Verification items for the finished model (mm, model axes). Face numbers are marked on the shaded views. Round coordinates to 2 decimals unless told otherwise and drop trailing zeros. Write each loop counter-clockwise with the first axis right and the second up, starting at its lowest first coordinate (ties: lowest second). Pieces come first, ordered by that corner, then holes.
from build123d import *

# Parameters (mm, degrees)
SKETCH_1_R      = 12
SKETCH_1_R_2    = 1.7
SKETCH_1_R_3    = 1.6
EXTRUDE_1_DEPTH = 2
SKETCH_2_R      = 2.5
EXTRUDE_2_DEPTH = 15


with BuildPart() as part:
    # 草图1 → 凸台-拉伸1 (new body)
    with BuildSketch(Plane(origin=(0, 0, 0), x_dir=(1, 0, 0), z_dir=(0, 1, 0))):
        Circle(SKETCH_1_R)
        with Locations((-8, 0)):
            Circle(SKETCH_1_R_2, mode=Mode.SUBTRACT)
        with Locations((0, 8)):
            Circle(SKETCH_1_R_3, mode=Mode.SUBTRACT)
        with Locations((8, 0)):
            Circle(SKETCH_1_R_2, mode=Mode.SUBTRACT)
        with Locations((0, -8)):
            Circle(SKETCH_1_R_3, mode=Mode.SUBTRACT)
    extrude(amount=EXTRUDE_1_DEPTH)

    # 草图2 → 凸台-拉伸2 (add)
    with BuildSketch(Plane(origin=(0, 2, 0), x_dir=(1, 0, 0), z_dir=(0, 1, 0))):
        Circle(SKETCH_2_R)
    extrude(amount=EXTRUDE_2_DEPTH)


solid = part.part
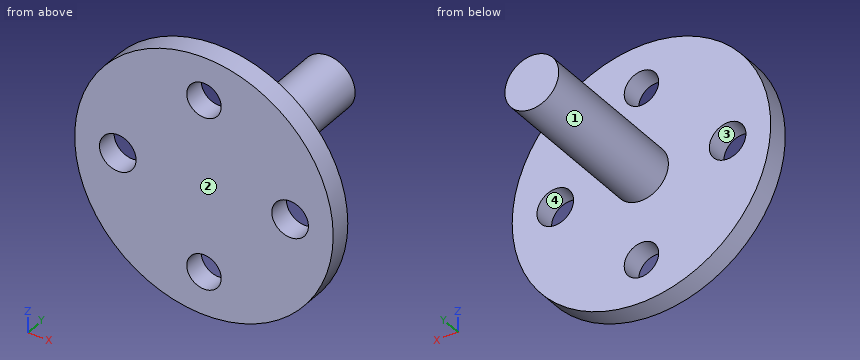
Q1. Release check for a two-part mould opening along Z. For the marked faces 1, 2, 3 and 4 record: released by +Z, released by -Z, zero draft, split by the parting line, or undercut.
Recorded:
face 1: split by the parting line
face 2: zero draft
face 3: undercut
face 4: undercut
Q2. Sectioned sample at D-D (z = -8). Enter the section's corners in (x, y), plus the area to 3 significant figures.
Recorded:
outline: (-8.94, 0) - (-1.6, 0) - (-1.6, 2) - (-8.94, 2) - close; (1.6, 0) - (8.94, 0) - (8.94, 2) - (1.6, 2) - close
area: 29.4 mm2
Q3. Material ranges on line 1 along X through (y, z) = (1.55, 0); line 2 along Z through (x, y) = (0, 1.35); line 3 along Z through (x, y) = (0.5, 1), recorded low to high.
Recorded:
line 1: x = -12 to -9.7, -6.3 to 6.3, 9.7 to 12
line 2: z = -12 to -9.6, -6.4 to 6.4, 9.6 to 12
line 3: z = -11.99 to -9.52, -6.48 to 6.48, 9.52 to 11.99
Q4. Sectioned sample at B-B (z = -0.5). Enter the section's corners in (x, y), plus the area to 3 significant figures.
Recorded:
outline: (-11.99, 0) - (-9.62, 0) - (-9.62, 2) - (-11.99, 2) - close; (-6.38, 0) - (6.38, 0) - (6.38, 2) - (2.45, 2) - (2.45, 17) - (-2.45, 17) - (-2.45, 2) - (-6.38, 2) - close; (9.62, 0) - (11.99, 0) - (11.99, 2) - (9.62, 2) - close
area: 108 mm2
Q5. Depth check by flat-ended pin: P1, Ø1, axis at x = -7, z = -3.5, coming from the -Y side; P2, Ø4, axis at y = 2.5, z = 2.5, coming from the +X side; P3, Ø1.5, axis at x = -1.5, z = -7.5, coming from the +Y side; P4, Ø5, axis at x = 3.5, y = 11, coming from the -Z side. Enter the tip coordinate at first touch or a pass-through.
Recorded:
P1: stops at y = 0
P2: stops at x = 11.99
P3: stops at y = 2
P4: stops at z = -2.29
Q6. Sectioned sample at A-A (x = 0). Enter the section's corners in (y, z), plus the area to 3 significant figures.
Recorded:
outline: (0, -12) - (2, -12) - (2, -9.6) - (0, -9.6) - close; (0, -6.4) - (2, -6.4) - (2, -2.5) - (17, -2.5) - (17, 2.5) - (2, 2.5) - (2, 6.4) - (0, 6.4) - close; (0, 9.6) - (2, 9.6) - (2, 12) - (0, 12) - close
area: 110 mm2
Q7. Sectioned sample at C-C (x = 8). Enter the section's corners in (y, z).
Recorded:
outline: (0, -8.94) - (2, -8.94) - (2, -1.7) - (0, -1.7) - close; (0, 1.7) - (2, 1.7) - (2, 8.94) - (0, 8.94) - close
